```python
from build123d import *

# Parameters (mm, degrees)
SKETCH2_W               = 40
SKETCH2_H               = 40
SKETCH2_R               = 1.6
SKETCH2_R_2             = 7
BOSS_EXTRUDE1_DEPTH     = 3
SKETCH3_W               = 43
SKETCH3_H               = 3
BOSS_EXTRUDE2_DEPTH     = 40
CUT_EXTRUDE1_DEPTH      = 72.056315694
CUT_EXTRUDE1_DEPTH_BACK = 72.056315694
SKETCH4_R               = 1.6
SKETCH4_R_2             = 4


with BuildPart() as part:
    # Sketch2 → Boss-Extrude1 (new body)
    with BuildSketch(Plane.XY):
        with Locations((20, -20)):
            Rectangle(SKETCH2_W, SKETCH2_H)
        with Locations((4.5, -20)):
            Circle(SKETCH2_R, mode=Mode.SUBTRACT)
        with Locations(Location((35.5, -20, 0), (0, 0, 180))):
            Circle(SKETCH2_R, mode=Mode.SUBTRACT)
        with Locations((12.25, -6.576606241)):
            Circle(SKETCH2_R, mode=Mode.SUBTRACT)
        with Locations(Location((27.75, -6.576606241, 0), (0, 0, 180))):
            Circle(SKETCH2_R, mode=Mode.SUBTRACT)
        with Locations((27.75, -33.423393759)):
            Circle(SKETCH2_R, mode=Mode.SUBTRACT)
        with Locations(Location((12.25, -33.423393759, 0), (0, 0, 180))):
            Circle(SKETCH2_R, mode=Mode.SUBTRACT)
        with Locations((20, -27)):
            Circle(SKETCH2_R_2, mode=Mode.SUBTRACT)
    extrude(amount=BOSS_EXTRUDE1_DEPTH)

    # Sketch3 → Boss-Extrude2 (add)
    with BuildSketch(Plane(origin=(0, 0, 0), x_dir=(0, 0, -1), z_dir=(1, 0, 0))):
        with Locations((-21.5, -41.5)):
            Rectangle(SKETCH3_W, SKETCH3_H)
    extrude(amount=BOSS_EXTRUDE2_DEPTH)

    # Sketch4 → Cut-Extrude1 (cut, two sides: drawn at the far end of the back side and taken through both)
    with BuildSketch(Plane(origin=(0, -40, 0), x_dir=(1, 0, 0), z_dir=(0, 1, 0)).offset(-CUT_EXTRUDE1_DEPTH_BACK)):
        with Locations(Location((9.393398282, -33.606601718, 0), (0, 0, 270))):
            Circle(SKETCH4_R)
        with Locations(Location((20, -23, 0), (0, 0, 270))):
            Circle(SKETCH4_R_2)
        with Locations(Location((9.393398282, -12.393398282, 0), (0, 0, 270))):
            Circle(SKETCH4_R)
        with Locations(Location((30.606601718, -12.393398282, 0), (0, 0, 270))):
            Circle(SKETCH4_R)
        with Locations(Location((30.606601718, -33.606601718, 0), (0, 0, 270))):
            Circle(SKETCH4_R)
    extrude(amount=CUT_EXTRUDE1_DEPTH + CUT_EXTRUDE1_DEPTH_BACK, mode=Mode.SUBTRACT)


solid = part.part
```
Design review of the part built by this model. Coordinates are the model's own, in mm. A direction names the side the tool comes from. Coordinates: 2 decimals unless noted, no trailing zeros. Order: outer loops, then holes, each group sorted by start corner. A loop starts at its lowest first (then second) coordinate and runs counter-clockwise, first axis right, second up. Notation, with made-up numbers: (35.25, 8) - (86.25, 8) arc R9 ccw to (86.25, 14) - close; hole circle Ø6 at (26, -12). An arc over 180 degrees is marked (long way). One line per question, with ' | ' between items.
Q1. Consider section D-D, the plane x = 20. Give the boundary of the cut face in (y, z).
Answer key:
outline: (-43, 0) - (-34, 0) - (-34, 3) - (-40, 3) - (-40, 19) - (-43, 19) - close; (-43, 27) - (-40, 27) - (-40, 43) - (-43, 43) - close; (-20, 0) - (0, 0) - (0, 3) - (-20, 3) - close
Q2. To check wall thickness, follow line 1 along Y through (x, z) = (35.5, 1.4); line 2 along Y through (x, z) = (33.5, 22.5); line 3 along Z through (x, y) = (37.5, -2). State the ranges of each line that lie inside material, in increasing order.
Answer key:
line 1: y = -43 to -21.6, -18.4 to 0 | line 2: y = -43 to -40 | line 3: z = 0 to 3
Q3. For faces 1 (the flat face through (20, -40, 28)), 2 (the flat face through (20, -42, 43)), list the 3-axis set-ups (+Z, -Z, +X, -X, +Y, -Y) from which the entire face can be reached by the end or side of a thin tool; tool diameter is ignored.
Answer key:
face 1: +Z, +X, -X, +Y | face 2: +Z, +X, -X, +Y, -Y
Q4. Consider section C-C, the plane y = -30.5. Give the boundary of the cut face in (x, z).
Answer key:
outline: (0, 0) - (13.94, 0) - (13.94, 3) - (0, 3) - close; (26.06, 0) - (40, 0) - (40, 3) - (26.06, 3) - close
Q5. Clearance check with flat-ended pins moving along their axes: pin 1 Ø8 at (x, z) = (9, 25) entering from +Y; pin 2 Ø5 at (x, y) = (4.5, -20) entering from +Z. State where each tip first meets the part, or that it passes through.
Answer key:
pin 1: stops at y = -40 | pin 2: stops at z = 3
Q6. Consider section B-B, the plane z = 13. Give the boundary of the cut face in (x, y).
Answer key:
outline: (0, -43) - (7.91, -43) - (7.91, -40) - (0, -40) - close; (10.87, -43) - (29.13, -43) - (29.13, -40) - (10.87, -40) - close; (32.09, -43) - (40, -43) - (40, -40) - (32.09, -40) - close
Q7. Consider section A-A, the plane x = 27.75. Give the boundary of the cut face in (y, z).
Answer key:
outline: (-43, 0) - (-35.02, 0) - (-35.02, 3) - (-40, 3) - (-40, 43) - (-43, 43) - close; (-31.82, 0) - (-8.18, 0) - (-8.18, 3) - (-31.82, 3) - close; (-4.98, 0) - (0, 0) - (0, 3) - (-4.98, 3) - close
Q8. The part is to be moulded in two halves that separate along X. For faces 3 (the flat face through (20, -17, 0)), 4 (the cylindrical face through (4.292, -18.414, 1.479)), 5 (the flat face through (0, -41, 12)), say which applies: +X half, -X half, draft (parallel to the pull), parting line (faces both ways), or undercut.
Answer key:
face 3: draft | face 4: undercut | face 5: -X half
